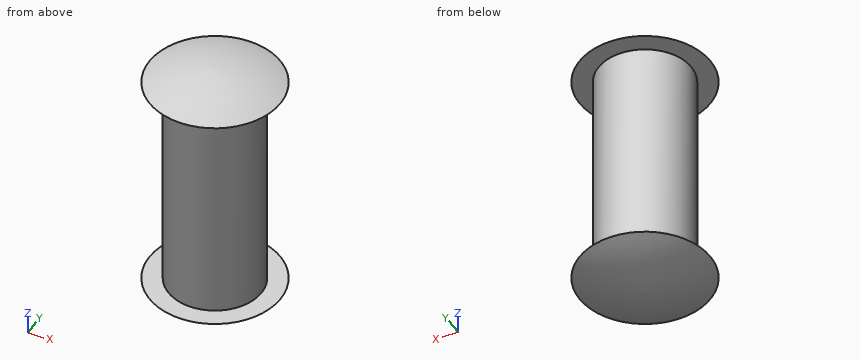
Autodesk Inventor part; units mm, degrees
ref_plane "YZ Plane" through (0, 0, 0) normal (1, 0, 0) x (0, 1, 0)
ref_plane "XZ Plane" through (0, 0, 0) normal (0, 1, 0) x (-1, 0, 0)
ref_plane "XY Plane" through (0, 0, 0) normal (0, 0, 1) x (1, 0, 0)
sketch "Sketch2" plane through (0, 0, 0) normal (0, 0, 1) x (1, 0, 0)
  circle A0 centre (0, 0) radius 1.25
  dimension "d44" = 2.5
extrude "Extrusion8" add sketch "Sketch2" along normal mid plane 6
sketch "Sketch3" plane through (0, 0, 3) normal (0, 0, 1) x (1, 0, 0)
  circle A0 centre (0, 0) radius 1.75
  dimension "d47" = 3.5
sketch "Sketch4" plane through (0, 0, 0) normal (0, 1, 0) x (-1, 0, 0)
  line L0 (1.25, 3) -> (-1.25, 3)
  line L1 (0, 3) -> (0, 3.4)
  arc A0 (0, 3.4) -> (-1.761, 3) centre (0.2088, -1.5956) ccw
  line L2 (0, 3) -> (-1.761, 3)
  point P0 (0, 0)
  dimension "d48" = 0.4
  dimension "d49" = 5
revolve "Revolution1" add sketch "Sketch4" angle 360 about axis through (0, 0, 3) along (0, 0, 1)
mirror "Mirror1" about plane through (0, 0, 0) normal (0, 0, 1) of "Revolution1"
properties part number "link7" material "Aluminum 6061"
Model file for the job. Use its own axes, mm. Coordinates: 2 decimals unless noted, no trailing zeros. Loops run counter-clockwise (first coordinate to the right, second up) from the corner with the lowest first, then second, coordinate; pieces in that order, holes last. Notation, with made-up numbers: (79.25, 12.25) - (100.25, 12.25) arc R18 ccw to (100.25, 21.25) - close; hole circle Ø5 at (-13, 77). An arc over 180 degrees is marked (long way). Answer as a JSON object with one key per item and string values. Group by question number.
(1) Cut at A-A (z = -0.5). Give the cut face in (x, y), then the cut area to 3 significant figures.
(2) Probe line 1 along Y through (x, z) = (0.35, -1.5); line 2 along Z through (x, y) = (-0.55, -0.95); line 3 along Z through (x, y) = (-0.1, 0.85). List the from-to ranges inside material, lowest first.
(3) Flat gauge pins, fed straight in: pin 1 (1.1 mm diameter, centred on x = 0.5, y = 0.5, fed in from +Z); pin 2 (1 mm diameter, centred on y = 0, z = -1.5, fed in from +X); pin 3 (1.5 mm diameter, centred on x = -0.5, z = 1.5, fed in from +Y). Where does each tip first touch, or does it go through?
Geometry says:
{
 "1": {"outline": "circle Ø2.5 at (0, 0)", "area": "4.91 mm^2"},
 "2": {"line 1": "y = -1.2 to 1.2", "line 2": "z = -3.23 to 3.23", "line 3": "z = -3.29 to 3.29"},
 "3": {"pin 1": "stops at z = 3.39", "pin 2": "stops at x = 1.25", "pin 3": "stops at y = 1.25"}
}
